```python
from build123d import *

# Parameters (mm, degrees)
F1_DEPTH = 25
F2_W     = 250
F2_H     = 20
F3_DEPTH = 20
F4_W     = 6.5
F4_H     = 10.5
F5_DEPTH = 100
F6_W     = 28.428983
F6_H     = 14.421839
F7_DEPTH = 20


with BuildPart() as f1:
    # F0 (on Right) → F1 (new body)
    with BuildSketch(Plane.YZ):
        Polygon((-17.320508, 0), (17.320508, 0), (34.641016, 30), (17.320508, 60), (-17.320508, 60), (-34.641016, 30), align=None)
    extrude(amount=F1_DEPTH)

    # F2 (on Top) → F3 (join)
    with BuildSketch(Plane.XY):
        with Locations((-125, 0)):
            Rectangle(F2_W, F2_H)
    extrude(amount=F3_DEPTH)

    # F4 (on face) → F5 (cut)
    with BuildSketch(Plane.XY.offset(20)):
        with Locations((-10, 0)):
            Rectangle(F4_W, F4_H)
        with Locations((-22, 0)):
            Rectangle(F4_W, F4_H)
        with Locations((-34, 0)):
            Rectangle(F4_W, F4_H)
        with Locations((-46, 0)):
            Rectangle(F4_W, F4_H)
        with Locations((-58, 0)):
            Rectangle(F4_W, F4_H)
        with Locations((-70, 0)):
            Rectangle(F4_W, F4_H)
        with Locations((-82, 0)):
            Rectangle(F4_W, F4_H)
        with Locations((-94, 0)):
            Rectangle(F4_W, F4_H)
        with Locations((-106, 0)):
            Rectangle(F4_W, F4_H)
        with Locations((-118, 0)):
            Rectangle(F4_W, F4_H)
        with Locations((-130, 0)):
            Rectangle(F4_W, F4_H)
        with Locations((-142, 0)):
            Rectangle(F4_W, F4_H)
        with Locations((-154, 0)):
            Rectangle(F4_W, F4_H)
        with Locations((-166, 0)):
            Rectangle(F4_W, F4_H)
        with Locations((-178, 0)):
            Rectangle(F4_W, F4_H)
        with Locations((-190, 0)):
            Rectangle(F4_W, F4_H)
        with Locations((-202, 0)):
            Rectangle(F4_W, F4_H)
        with Locations((-214, 0)):
            Rectangle(F4_W, F4_H)
        with Locations((-226, 0)):
            Rectangle(F4_W, F4_H)
        with Locations((-238, 0)):
            Rectangle(F4_W, F4_H)
    extrude(amount=-F5_DEPTH, mode=Mode.SUBTRACT)

    # F6 (on Top) → F7 (join)
    with BuildSketch(Plane.XY):
        with Locations((-14.214491, 0.158192)):
            Rectangle(F6_W, F6_H)
    extrude(amount=F7_DEPTH)


solid = f1.part
```
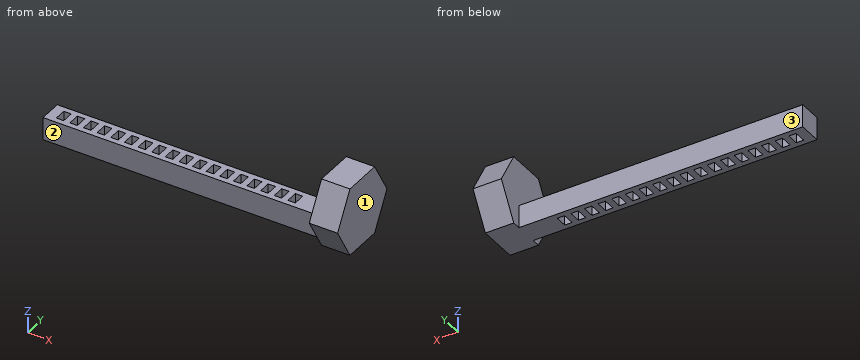
For this review, take the finished solid that the model builds, in its own axes (mm). Face numbers are marked on the shaded views. A direction names the side the tool comes from. Give positions to 0.01 mm unless a question says otherwise; leave off trailing zeros. Write each loop counter-clockwise with the first axis right and the second up, starting at its lowest first coordinate (ties: lowest second). Pieces come first, ordered by that corner, then holes. Notation, with made-up numbers: M -7,53.5 L 18,53.5 A27 ccw 18,87.5 Z; hole C 46,83.5 d6. An arc over 180 degrees is marked long. Answer as a JSON object with one key per item and string values. Group by question number.
Item 1: Consider section A-A on y = -0.5. Count the separate pieces of the cut face and the enclosed holes in it, plus the area to 3 significant figures.
Item 2: For probe 1 along X at (y, z) = (15, 16); probe 2 along Z at (x, y) = (-80, -7.5); probe 3 along Y at (x, z) = (-207.5, 12), list the stretches that pass through material, from the lowest coordinate up. Write a range as [from, to].
Item 3: Consider section B-B on x = -15. Write out the cut boundary in (y, z).
Item 4: For pin 1 Ø2 at (x, z) = (-119.5, 8) entering from -Y; pin 2 Ø7 at (x, z) = (-141, 12.5) entering from +Y; pin 3 Ø1 at (x, y) = (-113.5, 11) entering from +Z; pin 4 Ø4 at (y, z) = (2.5, 38) entering from -X, all flat-tipped, find the tip position at first contact; note any pin that passes through.
Item 5: Tool access review of the marked faces 1, 2 and 3: name each direction out of +Z, -Z, +X, -X, +Y, -Y from which nothing blocks a thin tool from reaching the whole face with its end or side.
Item 6: Consider section C-C on y = 15. Write out the cut boundary in (x, z).
Check result:
{
 "1": {"separate pieces": "19", "enclosed holes": "0", "area": "4,160 mm^2"},
 "2": {"probe 1": "x = [0, 25]", "probe 2": "z = [0, 20]", "probe 3": "y = [-10, 10]"},
 "3": {"outline": "M -10,0 L 10,0 L 10,20 L -10,20 Z"},
 "4": {"pin 1": "stops at y = -10", "pin 2": "stops at y = 10", "pin 3": "passes through", "pin 4": "stops at x = 0"},
 "5": {"face 1": "+Z, -Z, +X, +Y, -Y", "face 2": "+Z, -Z, -X, -Y", "face 3": "+Z, -Z, -X, +Y"},
 "6": {"outline": "M 0,0 L 25,0 L 25,60 L 0,60 Z"}
}
